Read the model definition and answer for the solid it produces. Units are mm, in the model's axes. A direction names the side the tool comes from. Coordinates: 2 decimals unless noted, no trailing zeros. Write each loop counter-clockwise with the first axis right and the second up, starting at its lowest first coordinate (ties: lowest second). Pieces come first, ordered by that corner, then holes. Notation, with made-up numbers: (12, 15) -> (62, 15) arc R18 cw to (62, 28) -> close; hole circle Ø11 at (50.25, 64.5). An arc over 180 degrees is marked (long way). Return JSON: item names as keys, results as strings.
Autodesk Inventor part; units mm, degrees
ref_plane "YZ Plane" through (0, 0, 0) normal (1, 0, 0) x (0, 1, 0)
ref_plane "XZ Plane" through (0, 0, 0) normal (0, 1, 0) x (-1, 0, 0)
ref_plane "XY Plane" through (0, 0, 0) normal (0, 0, 1) x (1, 0, 0)
sketch "Sketch1" plane through (0, 0, 0) normal (1, 0, 0) x (0, 1, 0)
  line L0 (0, 0) -> (50.8, 0)
  line L1 (50.8, 0) -> (50.8, -25.4)
  line L2 (50.8, -25.4) -> (0, -25.4)
  line L3 (0, -25.4) -> (0, 0)
  line L4 (3.175, -3.175) -> (47.625, -3.175)
  line L5 (47.625, -3.175) -> (47.625, -22.225)
  line L6 (47.625, -22.225) -> (3.175, -22.225)
  line L7 (3.175, -22.225) -> (3.175, -3.175)
  dimension "d0" = 50.8
  dimension "d1" = 25.4
  dimension "d2" = 44.45
  dimension "d3" = 19.05
  dimension "d4" = 3.175
  dimension "d5" = 3.175
extrude "Extrusion1" add sketch "Sketch1" along normal blind 711.2
sketch "Sketch2" plane through (0, 0, 0) normal (0, 0, 1) x (1, 0, 0)
  line L0 (0, 0) -> (0, 50.8)
  line L1 (0, 0) -> (711.2, 0)
  line L2 (711.2, 50.8) -> (711.2, 0)
  line L3 (0, 50.8) -> (711.2, 50.8)
  point P0 (31.75, 25.4)
  point P1 (679.45, 25.4)
  dimension "d8" = 31.75
  dimension "d9" = 25.4
  dimension "d10" = 31.75
  dimension "d11" = 25.4
hole "Hole3" at (31.75, 25.4, 0) at (679.45, 25.4, 0) direction (0, 0, -1) diameter 6.35 end through all
sketch "Sketch3" plane through (0, 0, 0) normal (0, 0, 1) x (1, 0, 0)
  circle A0 centre (31.75, 25.4) radius 3.175
  circle A1 centre (679.45, 25.4) radius 3.175
  line L0 (0, 0) -> (0, 50.8)
  line L1 (0, 0) -> (711.2, 0)
  line L2 (711.2, 50.8) -> (711.2, 0)
  line L3 (0, 50.8) -> (711.2, 50.8)
  point P0 (95.25, 25.4)
  point P1 (615.95, 25.4)
  dimension "d37" = 95.25
  dimension "d38" = 25.4
  dimension "d39" = 25.4
  dimension "d40" = 95.25
hole "Hole4" at (95.25, 25.4, 0) at (615.95, 25.4, 0) direction (0, 0, -1) diameter 6.35 end through all
properties part number "frame_wide"
1. The part is cut by section B-B (y = 39.5). Determine the outline of the cut face in (x, z) (3 decimals), then the cut area to 3 significant figures.
Taken from the geometry:
{"outline": "(0, -25.4) -> (711.2, -25.4) -> (711.2, -22.225) -> (0, -22.225) -> close; (0, -3.175) -> (711.2, -3.175) -> (711.2, 0) -> (0, 0) -> close", "area": "4,520 mm2"}
2. The part is cut by section A-A (z = -8.25). Determine the outline of the cut face in (x, y) (3 decimals).
Taken from the geometry:
{"outline": "(0, 0) -> (711.2, 0) -> (711.2, 3.175) -> (0, 3.175) -> close; (0, 47.625) -> (711.2, 47.625) -> (711.2, 50.8) -> (0, 50.8) -> close"}
3. Consider L1, parallel to X at y = 25.4, z = -23.25 (3 decimals); L2, parallel to Z at x = 115.5, y = 30.5 (3 decimals); L3, parallel to Y at x = 329, z = -8.25 (3 decimals). Determine where each line is inside the solid, lowest interval first.
Taken from the geometry:
{"L1": "x = 0 to 28.575, 34.925 to 92.075, 98.425 to 612.775, 619.125 to 676.275, 682.625 to 711.2", "L2": "z = -25.4 to -22.225, -3.175 to 0", "L3": "y = 0 to 3.175, 47.625 to 50.8"}
4. For a pull along Y with two mould halves and no side action, classify faces 1 (the face through (351, 26, -25.4)), 2 (the face through (351, 0, -13)), 3 (the face through (351, 26, -22.225)), 4 (the face through (351, 25, -3.175)) as +Y half, -Y half, draft (parallel to the pull), parting line (faces both ways), or undercut.
Taken from the geometry:
{"face 1": "draft", "face 2": "-Y half", "face 3": "undercut", "face 4": "undercut"}
5. The part is cut by section C-C (x = 433.5). Determine the outline of the cut face in (y, z) (3 decimals), then the cut area to 3 significant figures.
Taken from the geometry:
{"outline": "(0, -25.4) -> (50.8, -25.4) -> (50.8, 0) -> (0, 0) -> close; hole (3.175, -22.225) -> (47.625, -22.225) -> (47.625, -3.175) -> (3.175, -3.175) -> close", "area": "444 mm2"}
6. A tool of negligible diameter and unlimited length cuts with its end or side. For faces 5 (the face through (351, 3.175, -13)), 6 (the face through (0, 25, -2)), from which of +Z, -Z, +X, -X, +Y, -Y can it reach the whole face along a straight path? Write none if from no direction.
Taken from the geometry:
{"face 5": "+X, -X", "face 6": "+Z, -Z, -X, +Y, -Y"}
